Check sheet for the modelled part. Datum: model origin and axes. Units: mm. Face numbers are marked on the shaded views. A direction names the side the tool comes from. Round coordinates to 2 decimals unless told otherwise and drop trailing zeros. Write each loop counter-clockwise with the first axis right and the second up, starting at its lowest first coordinate (ties: lowest second). Pieces come first, ordered by that corner, then holes. Notation, with made-up numbers: M 37,-3 L 61,-3 A15 ccw 61,13 Z; hole C 12.25,-5 d11. An arc over 180 degrees is marked long. One line per item, written item: value.
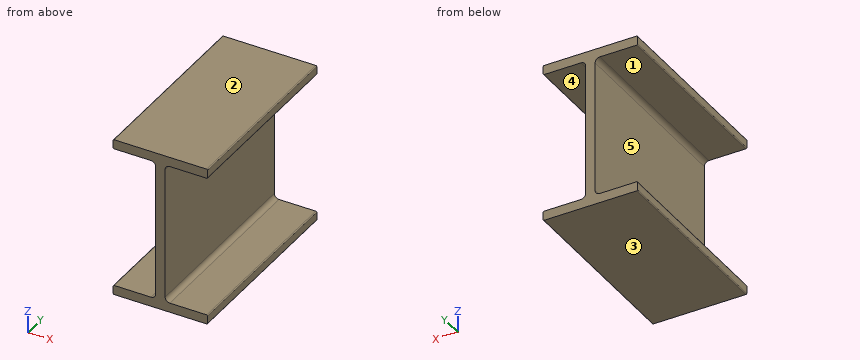
from build123d import *

# Parameters (mm, degrees)
F1_DEPTH = 50.8


with BuildPart() as f1:
    # F0 (on Front) → F1 (new body)
    with BuildSketch(Plane.XZ):
        with BuildLine():
            ThreePointArc((-12.7, 19.304), (-12.625605, 19.124395), (-12.446, 19.05))
            Line((-12.446, 19.05), (-2.54, 19.05))
            ThreePointArc((-2.54, 19.05), (-1.641974, 18.678026), (-1.27, 17.78))
            Line((-1.27, 17.78), (-1.27, -17.78))
            ThreePointArc((-1.27, -17.78), (-1.641974, -18.678026), (-2.54, -19.05))
            Line((-2.54, -19.05), (-12.446, -19.05))
            ThreePointArc((-12.446, -19.05), (-12.625605, -19.124395), (-12.7, -19.304))
            Line((-12.7, -19.304), (-12.7, -21.336))
            ThreePointArc((-12.7, -21.336), (-12.625605, -21.515605), (-12.446, -21.59))
            Line((-12.446, -21.59), (12.446, -21.59))
            ThreePointArc((12.446, -21.59), (12.625605, -21.515605), (12.7, -21.336))
            Line((12.7, -21.336), (12.7, -19.304))
            ThreePointArc((12.7, -19.304), (12.625605, -19.124395), (12.446, -19.05))
            Line((12.446, -19.05), (2.54, -19.05))
            ThreePointArc((2.54, -19.05), (1.641974, -18.678026), (1.27, -17.78))
            Line((1.27, -17.78), (1.27, 17.78))
            ThreePointArc((1.27, 17.78), (1.641974, 18.678026), (2.54, 19.05))
            Line((2.54, 19.05), (12.446, 19.05))
            ThreePointArc((12.446, 19.05), (12.625605, 19.124395), (12.7, 19.304))
            Line((12.7, 19.304), (12.7, 21.336))
            ThreePointArc((12.7, 21.336), (12.625605, 21.515605), (12.446, 21.59))
            Line((12.446, 21.59), (-12.446, 21.59))
            ThreePointArc((-12.446, 21.59), (-12.625605, 21.515605), (-12.7, 21.336))
            Line((-12.7, 21.336), (-12.7, 19.304))
        make_face()
    extrude(amount=F1_DEPTH)


solid = f1.part
Q1. Scan lines: line 1 (Z direction, x = -4, y = -11); line 2 (X direction, y = -34, z = -8); line 3 (Z direction, x = -1.75, y = -13). Record each from-to range of solid material in increasing order. Write a range as [from, to].
Completed:
line 1: [-21.59, -19.05], [19.05, 21.59]
line 2: [-1.27, 1.27]
line 3: [-21.59, -18.77], [18.77, 21.59]
Q2. Access from +Z, -Z, +X, -X, +Y, -Y to the whole of each face (thin tool, end or side, straight path). Record for the marked faces 4 and 5.
Completed:
face 4: +X, +Y, -Y
face 5: -X, +Y, -Y
Q3. Depth check by flat-ended pin: P1, Ø10.5, axis at y = -21.5, z = 2.5, coming from the +X side; P2, Ø10.5, axis at y = -34, z = -4, coming from the -X side. Enter the tip coordinate at first touch or a pass-through.
Completed:
P1: x = 1.27
P2: x = -1.27
Q4. Draft check along Z on the marked faces 1, 2 and 3. Enter one of: pulls with the +Z half, pulls with the -Z half, needs draft (parallel to the pull), parting line crosses it, or undercut.
Completed:
face 1: undercut
face 2: pulls with the +Z half
face 3: pulls with the -Z half
Q5. Sectioned sample at C-C on z = 5.5. Enter the section's corners in (x, y).
Completed:
outline: M -1.27,-50.8 L 1.27,-50.8 L 1.27,0 L -1.27,0 Z
Q6. Sectioned sample at B-B on y = -36. Enter the section's corners in (x, z).
Completed:
outline: M -12.7,-21.34 A0.25 ccw -12.45,-21.59 L 12.45,-21.59 A0.25 ccw 12.7,-21.34 L 12.7,-19.3 A0.25 ccw 12.45,-19.05 L 2.54,-19.05 A1.27 cw 1.27,-17.78 L 1.27,17.78 A1.27 cw 2.54,19.05 L 12.45,19.05 A0.25 ccw 12.7,19.3 L 12.7,21.34 A0.25 ccw 12.45,21.59 L -12.45,21.59 A0.25 ccw -12.7,21.34 L -12.7,19.3 A0.25 ccw -12.45,19.05 L -2.54,19.05 A1.27 cw -1.27,17.78 L -1.27,-17.78 A1.27 cw -2.54,-19.05 L -12.45,-19.05 A0.25 ccw -12.7,-19.3 Z
Q7. Sectioned sample at A-A on x = -4.5. Enter the section's corners in (y, z).
Completed:
outline: M -50.8,-21.59 L 0,-21.59 L 0,-19.05 L -50.8,-19.05 Z; M -50.8,19.05 L 0,19.05 L 0,21.59 L -50.8,21.59 Z
